Could you check a few things on this model? Use its own coordinates, in mm. A direction names the side the tool comes from. Round coordinates to 2 decimals unless told otherwise and drop trailing zeros. Write each loop counter-clockwise with the first axis right and the second up, starting at its lowest first coordinate (ties: lowest second). Pieces come first, ordered by that corner, then holes. Notation, with made-up numbers: M -15.75,85 L -11.75,85 A14 cw -11.75,92 Z; hole C 33.25,-39 d11. An arc over 180 degrees is marked long. One line per item, written item: value. Start each with the question number.
(1) I'm going to push flat-ended pins straight in: pin 1 Ø0.8 at (x, z) = (2, -38.5) entering from +Y; pin 2 Ø1.5 at (x, z) = (1.5, 9.5) entering from +Y; pin 3 Ø0.8 at (x, z) = (1.5, 38.5) entering from +Y. Where does each tip first touch, or does it pass through?
(2) If I drill on L1, parallel to Z at x = 1, y = 35.5; L2, parallel to Y at x = 0.25, z = -22; L3, parallel to Y at x = 0.7, z = -28.5, over which ranges is the centre line in solid material (lowest first)?
(3) I want a section at B-B on z = 24. Please give me the cut outline in (x, y).
(4) Which directions (+Z, -Z, +X, -X, +Y, -Y) give clear straight access to the entire face, cutting with the end or side of a thin tool? Please do faces 1 (the face through (1, 97, -37.3)), 2 (the face through (1, -1, 13.5)), 3 (the face through (1, 85, -39)), 4 (the face through (1, 45, 39)).
(5) Thinking about a two-plate mould opening in Y: for faces 5 (the face through (1, -1, -22.5)), 6 (the face through (1, 55, -39)), 7 (the face through (1.369, 64.875, 15.6)), which applies, released by +Y, released by -Y, zero draft, split by the parting line, or undercut?
(6) I want a section at A-A on y = 58.5. Please give me the cut outline in (x, z), and give its area (3 significant figures).
```python
from build123d import *

# Parameters (mm, degrees)
BOSS_EXTRU_1_DEPTH              = 2.7
ESQUISSE2_W                     = 9
ESQUISSE2_H                     = 2.7
BOSS_EXTRU_2_DEPTH              = 2.7
R_P_TITION_LIN_AIRE1_COUNT      = 3
R_P_TITION_LIN_AIRE1_PITCH      = 18
R_P_TITION_LIN_AIRE1_COL_COUNT  = 2
R_P_TITION_LIN_AIRE1_COL_PITCH  = 18
ESQUISSE3_W                     = 2.7
ESQUISSE3_H                     = 10
BOSS_EXTRU_3_DEPTH              = 2.7
R_P_TITION_LIN_AIRE2_COUNT      = 5
R_P_TITION_LIN_AIRE2_PITCH      = 20
R_P_TITION_LIN_AIRE2_COUNT_DIR2 = 2
R_P_TITION_LIN_AIRE2_PITCH_DIR2 = 77.3
CONG_1_R                        = 40


with BuildPart() as part:
    # Esquisse1 → Boss.-Extru.1 (new body)
    with BuildSketch(Plane(origin=(0, 0, 0), x_dir=(0, 0, -1), z_dir=(1, 0, 0))):
        Polygon((37.3, 100), (13.3, 100), (-13.3, 60), (-37.3, 60), (-37.3, 0), (37.3, 0), align=None)
    extrude(amount=BOSS_EXTRU_1_DEPTH)

    # Esquisse2 → Boss.-Extru.2 (add)
    with BuildSketch(Plane(origin=(0, 0, 0), x_dir=(0, 0, -1), z_dir=(1, 0, 0))):
        with Locations((-9, -1.35)):
            Rectangle(ESQUISSE2_W, ESQUISSE2_H)
    boss_extru_2 = extrude(amount=BOSS_EXTRU_2_DEPTH)

    # Répétition linéaire1: Boss.-Extru.2 ×3
    with Locations(*[(0, 0, -i * R_P_TITION_LIN_AIRE1_PITCH) for i in range(1, R_P_TITION_LIN_AIRE1_COUNT)]):
        add(boss_extru_2)

    # Répétition linéaire1 col: Boss.-Extru.2 ×2
    with Locations(*[(0, 0, i * R_P_TITION_LIN_AIRE1_COL_PITCH) for i in range(1, R_P_TITION_LIN_AIRE1_COL_COUNT)]):
        add(boss_extru_2)

    # Esquisse3 → Boss.-Extru.3 (add)
    with BuildSketch(Plane(origin=(0, 0, 0), x_dir=(0, 0, -1), z_dir=(1, 0, 0))):
        with Locations((-38.65, 10)):
            Rectangle(ESQUISSE3_W, ESQUISSE3_H)
    boss_extru_3 = extrude(amount=BOSS_EXTRU_3_DEPTH)

    # Répétition linéaire2: Boss.-Extru.3 5 × 2, 2 skipped
    with Locations(*[(0, i * R_P_TITION_LIN_AIRE2_PITCH, -j * R_P_TITION_LIN_AIRE2_PITCH_DIR2) for i in range(R_P_TITION_LIN_AIRE2_COUNT) for j in range(R_P_TITION_LIN_AIRE2_COUNT_DIR2) if (i, j) not in ((0, 0), (3, 0), (4, 0))]):
        add(boss_extru_3)

    # Congé1
    cong_1_edges = [part.edges().sort_by_distance(p)[0] for p in [
        (1.35, 60, 13.3),
        (1.35, 100, -13.3),
    ]]
    fillet(cong_1_edges, radius=CONG_1_R)


solid = part.part
```
Found:
1. pin 1: stops at y = 95
1. pin 2: stops at y = 69.59
1. pin 3: stops at y = 55
2. L1: z = -37.3 to 37.3
2. L2: y = 0 to 97.92
2. L3: y = -2.7 to 99.51
3. outline: M 0,-2.7 L 2.7,-2.7 L 2.7,61.47 L 0,61.47 Z
4. face 1: -Z, +X, -X, +Y
4. face 2: +X, -X, -Y
4. face 3: -Z, +X, -X
4. face 4: +Z, +X, -X
5. face 5: zero draft
5. face 6: undercut
5. face 7: released by +Y
6. outline: M 0,-37.3 L 2.7,-37.3 L 2.7,37.3 L 0,37.3 Z
6. area: 201 mm²
